Could you check a few things on this model? Use its own coordinates, in mm. A direction names the side the tool comes from. Round coordinates to 2 decimals unless told otherwise and drop trailing zeros. Loops run counter-clockwise (first coordinate to the right, second up) from the corner with the lowest first, then second, coordinate; pieces in that order, holes last. Notation, with made-up numbers: (21.5, 37.5) -> (80.5, 37.5) arc R24 cw to (80.5, 73.5) -> close; hole circle Ø4 at (42, 4). An arc over 180 degrees is marked (long way). One line per item, written item: value.
from build123d import *

# Parameters (mm, degrees)
ESBO_O1_R                = 3
RESSALTO_EXTRUS_O1_DEPTH = 22


with BuildPart() as part:
    # Esboço1 → Ressalto-extrusão1 (new body)
    with BuildSketch(Plane.XY):
        with BuildLine():
            Line((-49.119135606, 68), (49.119135606, 68))
            ThreePointArc((49.119135606, 68), (54.543435225, 67.250375935), (59.56111629, 65.057697365))
            ThreePointArc((59.56111629, 65.057697365), (73.40190502, 57.827992781), (88.094517748, 52.539969306))
            Line((88.094517748, 52.539969306), (88.094517748, 47.321908149))
            ThreePointArc((88.094517748, 47.321908149), (75.969961031, 51.336342949), (64.340736461, 56.616655277))
            ThreePointArc((64.340736461, 56.616655277), (60.029722653, 57.739663923), (55.658771962, 56.878979006))
            ThreePointArc((55.658771962, 56.878979006), (52.268274515, 56.633748331), (49.504565952, 58.613022442))
            ThreePointArc((49.504565952, 58.613022442), (45.919841237, 61.796967806), (41.265094556, 62.946355775))
            Line((41.265094556, 62.946355775), (-41.265094556, 62.946355775))
            ThreePointArc((-41.265094556, 62.946355775), (-45.919841237, 61.796967806), (-49.504565952, 58.613022442))
            ThreePointArc((-49.504565952, 58.613022442), (-52.268274515, 56.633748331), (-55.658771962, 56.878979006))
            ThreePointArc((-55.658771962, 56.878979006), (-60.029722653, 57.739663923), (-64.340736461, 56.616655277))
            ThreePointArc((-64.340736461, 56.616655277), (-75.969961031, 51.336342949), (-88.094517748, 47.321908149))
            Line((-88.094517748, 47.321908149), (-88.094517748, 52.539969306))
            ThreePointArc((-88.094517748, 52.539969306), (-73.40190502, 57.827992781), (-59.56111629, 65.057697365))
            ThreePointArc((-59.56111629, 65.057697365), (-54.543435225, 67.250375935), (-49.119135606, 68))
        make_face()
        with Locations((-53.62430165, 61.446355775)):
            Circle(ESBO_O1_R, mode=Mode.SUBTRACT)
        with Locations((53.62430165, 61.446355775)):
            Circle(ESBO_O1_R, mode=Mode.SUBTRACT)
    extrude(amount=RESSALTO_EXTRUS_O1_DEPTH)


solid = part.part
(1) For faces 5 (the face through (56.5, 62.3, 10.8)), 6 (the face through (1, 62.946, 11)), which set-ups out of +Z, -Z, +X, -X, +Y, -Y let a thin tool reach every point of the face, with its end or its side?
Recorded:
face 5: +Z, -Z
face 6: +Z, -Z, -Y
(2) I'm going to push flat-ended pins straight in: pin 1 Ø8 at (x, y) = (53.62, 61.45) entering from +Z; pin 2 Ø8 at (y, z) = (60.5, 13.5) entering from +X; pin 3 Ø3 at (x, z) = (-64.5, 11) entering from +Y; pin 4 Ø12 at (x, z) = (36, 5) entering from -Y. Where does each tip first touch, or does it pass through?
Recorded:
pin 1: z = 22
pin 2: x = 76.56
pin 3: y = 63.03
pin 4: y = 62.92
(3) Thinking about a two-plate mould opening in Y: for faces 1 (the face through (-54.62, 67.23, 10.85)), 2 (the face through (-75.803, 51.402, 10.846)), 3 (the face through (-54.01, 64.42, 10.85)), 4 (the face through (-88.095, 50, 11)), which applies, released by +Y, released by -Y, zero draft, split by the parting line, or undercut?
Recorded:
face 1: released by +Y
face 2: released by -Y
face 3: undercut
face 4: zero draft
(4) If we section it at A-A, the plane z = 10.5: Please give me the cut outline in (x, y), then the cut area to 3 significant figures.
Recorded:
outline: (-88.09, 47.32) arc R120 ccw to (-64.34, 56.62) arc R10 cw to (-55.66, 56.88) arc R5 ccw to (-49.5, 58.61) arc R10 cw to (-41.27, 62.95) -> (41.27, 62.95) arc R10 cw to (49.5, 58.61) arc R5 ccw to (55.66, 56.88) arc R10 cw to (64.34, 56.62) arc R120 ccw to (88.09, 47.32) -> (88.09, 52.54) arc R115 cw to (59.56, 65.06) arc R20 ccw to (49.12, 68) -> (-49.12, 68) arc R20 ccw to (-59.56, 65.06) arc R115 cw to (-88.09, 52.54) -> close; hole circle Ø6 at (-53.62, 61.45); hole circle Ø6 at (53.62, 61.45)
area: 981 mm²
(5) If I drill on L1, parallel to X at y = 59, z = 11; L2, parallel to X at y = 59.25, z = 15.5; L3, parallel to Y at x = -28.5, z = 17.75, over which ranges is the centre line in solid material (lowest first)?
Recorded:
L1: -70.82 to -55.36, -51.89 to -49.22, 49.22 to 51.89, 55.36 to 70.82
L2: -70.29 to -55.67, -51.58 to -49.03, 49.03 to 51.58, 55.67 to 70.29
L3: 62.95 to 68
(6) If we section it at B-B, the plane x = -12: Please give me the cut outline in (y, z), then the cut area to 3 significant figures.
Recorded:
outline: (62.95, 0) -> (68, 0) -> (68, 22) -> (62.95, 22) -> close
area: 111 mm²
(7) If we section it at C-C, the plane x = -62: Please give me the cut outline in (y, z).
Recorded:
outline: (57.48, 0) -> (63.61, 0) -> (63.61, 22) -> (57.48, 22) -> close
